Can you work these out from the model? Positions are in its coordinate system, mm. Face numbers are marked on the shaded views. A direction names the side the tool comes from. Round coordinates to 2 decimals unless told otherwise and drop trailing zeros. Write each loop counter-clockwise with the first axis right and the second up, starting at its lowest first coordinate (ties: lowest second). Pieces come first, ordered by that corner, then holes. Notation, with made-up numbers: (56, 33) -> (73, 33) arc R16 ccw to (73, 55) -> close; hole circle Ø6 at (77.25, 4). An arc over 180 degrees is marked (long way). Use CSV: the item, a comma, the result in double quotes.
```python
from build123d import *

# Parameters (mm, degrees)
SALIENTE_EXTRUIR1_DEPTH      = 77.5
SALIENTE_EXTRUIR1_DEPTH_BACK = 77.5
CROQUIS3_W                   = 82.87
CROQUIS3_H                   = 362
CROQUIS4_W                   = 230
CROQUIS4_H                   = 315.74
CROQUIS4_R                   = 110
SALIENTE_EXTRUIR2_DEPTH      = 495.3
CORTAR_EXTRUIR1_DEPTH        = 447.936166471
CORTAR_EXTRUIR1_DEPTH_BACK   = 447.936166471
CROQUIS5_W                   = 42
CROQUIS5_H                   = 360
CROQUIS6_W                   = 140.888518715
CROQUIS6_H                   = 52
CROQUIS6_W_2                 = 161.625356967
CORTAR_EXTRUIR2_DEPTH        = 332
CORTAR_EXTRUIR3_START        = -495.3
CORTAR_EXTRUIR3_DEPTH        = 495.3
CROQUIS12_R                  = 9.525
CORTAR_EXTRUIR9_DEPTH        = 230
CROQUIS15_R                  = 14.29
CORTAR_EXTRUIR10_DEPTH       = 48
CORTAR_EXTRUIR11_START       = -48
CROQUIS16_R                  = 14.29
CORTAR_EXTRUIR11_DEPTH       = 48
CROQUIS18_W                  = 231.274148036
CROQUIS18_H                  = 332
CORTAR_EXTRUIR12_DEPTH       = 48
CROQUIS19_W                  = 231.274148036
CROQUIS19_H                  = 332
CORTAR_EXTRUIR13_DEPTH       = 48
CROQUIS20_W                  = 52.279992223
CROQUIS20_H                  = 50
CORTAR_EXTRUIR14_DEPTH       = 48
CROQUIS21_W                  = 52.279992223
CROQUIS21_H                  = 50
CORTAR_EXTRUIR15_DEPTH       = 48


with BuildPart() as part:
    # Croquis1 → Revolución1 (revolve)
    with BuildSketch(Plane.XY, mode=Mode.PRIVATE) as revoluci_n1_sk:
        Polygon((-110, 93.3), (-105, 93.3), (-51.5, 0), (-51.5, -362), (-105, -402), (-110, -402), align=None)
    revolve(revoluci_n1_sk.sketch.rotate(Axis((0, 0, 0), (0, 1, 0)), 270), axis=Axis((0, 0, 0), (0, 1, 0)))

    # Croquis3 → Saliente-Extruir1 (add, two sides: drawn at the far end of the back side and taken through both)
    with BuildSketch(Plane(origin=(0, 0, 0), x_dir=(0, 0, -1), z_dir=(1, 0, 0)).offset(-SALIENTE_EXTRUIR1_DEPTH_BACK)):
        with Locations((116.435, -181)):
            Rectangle(CROQUIS3_W, CROQUIS3_H)
        with Locations((-116.435, -181)):
            Rectangle(CROQUIS3_W, CROQUIS3_H)
    extrude(amount=SALIENTE_EXTRUIR1_DEPTH + SALIENTE_EXTRUIR1_DEPTH_BACK)

    # Croquis4 → Saliente-Extruir2 (add)
    with BuildSketch(Plane(origin=(0, 93.3, 0), x_dir=(1, 0, 0), z_dir=(0, 1, 0))):
        Rectangle(CROQUIS4_W, CROQUIS4_H)
        Circle(CROQUIS4_R, mode=Mode.SUBTRACT)
    extrude(amount=-SALIENTE_EXTRUIR2_DEPTH)

    # Croquis5 → Cortar-Extruir1 (cut, two sides: drawn at the far end of the back side and taken through both)
    with BuildSketch(Plane.XY.offset(-CORTAR_EXTRUIR1_DEPTH_BACK)):
        with Locations((0, -180)):
            Rectangle(CROQUIS5_W, CROQUIS5_H)
    extrude(amount=CORTAR_EXTRUIR1_DEPTH + CORTAR_EXTRUIR1_DEPTH_BACK, mode=Mode.SUBTRACT)

    # Croquis6 → Cortar-Extruir2 (cut)
    with BuildSketch(Plane(origin=(0, 0, 0), x_dir=(1, 0, 0), z_dir=(0, 1, 0))):
        with Locations((-100.594259358, -3)):
            Rectangle(CROQUIS6_W, CROQUIS6_H)
        with Locations((110.962678484, 3)):
            Rectangle(CROQUIS6_W_2, CROQUIS6_H)
    extrude(amount=-CORTAR_EXTRUIR2_DEPTH, mode=Mode.SUBTRACT)

    # Croquis7 → Cortar-Extruir3 (cut)
    with BuildSketch(Plane(origin=(0, 93.3, 0), x_dir=(1, 0, 0), z_dir=(0, 1, 0)).offset(CORTAR_EXTRUIR3_START)):
        Polygon((-115, 157.87), (-57.5, 157.87), (-57.5, 115.637074018), (-115, 53.01), align=None)
        Polygon((57.5, 115.637074018), (57.5, 157.87), (115, 157.87), (115, 53.01), align=None)
        Polygon((115, -157.87), (57.5, -157.87), (57.5, -115.637074018), (115, -53.01), align=None)
        Polygon((-57.5, -115.637074018), (-57.5, -157.87), (-115, -157.87), (-115, -53.01), align=None)
    extrude(amount=CORTAR_EXTRUIR3_DEPTH, mode=Mode.SUBTRACT)

    # Croquis12 → Cortar-Extruir9 (cut)
    with BuildSketch(Plane.ZY.offset(115)):
        with Locations(Location((-90.237074018, -327.07, 0), (0, 0, 90))):
            Circle(CROQUIS12_R)
        with Locations(Location((-90.237074018, -35.052, 0), (0, 0, 90))):
            Circle(CROQUIS12_R)
        with Locations(Location((90.237074018, -35.052, 0), (0, 0, 270))):
            Circle(CROQUIS12_R)
        with Locations(Location((90.237074018, -327.07, 0), (0, 0, 270))):
            Circle(CROQUIS12_R)
    extrude(amount=-CORTAR_EXTRUIR9_DEPTH, mode=Mode.SUBTRACT)

    # Croquis15 → Cortar-Extruir10 (cut)
    with BuildSketch(Plane.ZY.offset(115)):
        with Locations((-90.237074018, -35.052)):
            Circle(CROQUIS15_R)
        with Locations((90.237074018, -35.052)):
            Circle(CROQUIS15_R)
        with Locations((90.237074018, -327.07)):
            Circle(CROQUIS15_R)
        with Locations((-90.237074018, -327.07)):
            Circle(CROQUIS15_R)
    extrude(amount=-CORTAR_EXTRUIR10_DEPTH, mode=Mode.SUBTRACT)

    # Croquis16 → Cortar-Extruir11 (cut)
    with BuildSketch(Plane(origin=(115, 0, 0), x_dir=(0, 0, -1), z_dir=(1, 0, 0)).offset(CORTAR_EXTRUIR11_START)):
        with Locations(Location((-90.237074018, -35.052, 0), (0, 0, 180))):
            Circle(CROQUIS16_R)
        with Locations(Location((90.237074018, -35.052, 0), (0, 0, 180))):
            Circle(CROQUIS16_R)
        with Locations(Location((90.237074018, -327.07, 0), (0, 0, 180))):
            Circle(CROQUIS16_R)
        with Locations(Location((-90.237074018, -327.07, 0), (0, 0, 180))):
            Circle(CROQUIS16_R)
    extrude(amount=CORTAR_EXTRUIR11_DEPTH, mode=Mode.SUBTRACT)

    # Croquis18 → Cortar-Extruir12 (cut)
    with BuildSketch(Plane(origin=(115, 0, 0), x_dir=(0, 0, -1), z_dir=(1, 0, 0))):
        with Locations((0, -166)):
            Rectangle(CROQUIS18_W, CROQUIS18_H)
    extrude(amount=-CORTAR_EXTRUIR12_DEPTH, mode=Mode.SUBTRACT)

    # Croquis19 → Cortar-Extruir13 (cut)
    with BuildSketch(Plane.ZY.offset(115)):
        with Locations((0, -166)):
            Rectangle(CROQUIS19_W, CROQUIS19_H)
    extrude(amount=-CORTAR_EXTRUIR13_DEPTH, mode=Mode.SUBTRACT)

    # Croquis20 → Cortar-Extruir14 (cut)
    with BuildSketch(Plane.ZY.offset(115)):
        with Locations((-79.149996112, 25)):
            Rectangle(CROQUIS20_W, CROQUIS20_H)
        with Locations((79.149996112, 25)):
            Rectangle(CROQUIS20_W, CROQUIS20_H)
    extrude(amount=-CORTAR_EXTRUIR14_DEPTH, mode=Mode.SUBTRACT)

    # Croquis21 → Cortar-Extruir15 (cut)
    with BuildSketch(Plane(origin=(115, 0, 0), x_dir=(0, 0, -1), z_dir=(1, 0, 0))):
        with Locations((79.149996112, 25)):
            Rectangle(CROQUIS21_W, CROQUIS21_H)
        with Locations((-79.149996112, 25)):
            Rectangle(CROQUIS21_W, CROQUIS21_H)
    extrude(amount=-CORTAR_EXTRUIR15_DEPTH, mode=Mode.SUBTRACT)


solid = part.part
```
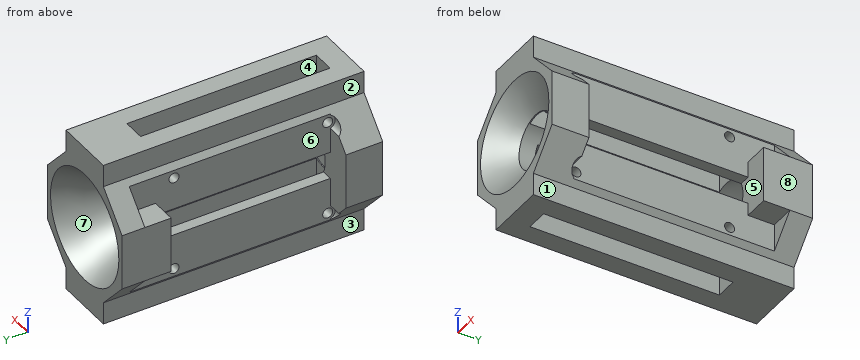
Q1. Suppose I cut it at A-A (y = -204.5). Write out the boundary of the cut face in (x, z).
Resolved:
outline,"(-67, -105.29) -> (-57.5, -115.64) -> (-57.5, -157.87) -> (-21, -157.87) -> (-21, -47.02) arc R51.5 cw to (-46.08, -23) -> (-67, -23) -> close; (-67, 29) -> (-42.56, 29) arc R51.5 cw to (-21, 47.02) -> (-21, 157.87) -> (-57.5, 157.87) -> (-57.5, 115.64) -> (-67, 105.29) -> close; (21, -157.87) -> (57.5, -157.87) -> (57.5, -115.64) -> (67, -105.29) -> (67, -29) -> (42.56, -29) arc R51.5 cw to (21, -47.02) -> close; (21, 47.02) arc R51.5 cw to (46.08, 23) -> (67, 23) -> (67, 105.29) -> (57.5, 115.64) -> (57.5, 157.87) -> (21, 157.87) -> close"
Q2. Will these pins go through, and if not, where does the flat tip stop? P1, Ø21, axis at y = -121, z = 143.5, coming from the +X side; P2, Ø8, axis at y = -90, z = 59.5, coming from the -X side; P3, Ø5, axis at x = 81.5, z = -28, coming from the -Y side.
Resolved:
P1,"stops at x = 57.5"
P2,"stops at x = -67"
P3,"stops at y = -389.79"
Q3. On a 3-axis mill with a long thin cutter (end or side, diameter ignored), from which of +Z, -Z, +X, -X, +Y, -Y can I reach the whole of each face in a straight line? I mean the marked faces 1, 2, 3, 4 and 5. Say none if no direction works.
Resolved:
face 1,"-Z, +X, +Y, -Y"
face 2,"+Z, -X, +Y, -Y"
face 3,"-Z, -X, +Y, -Y"
face 4,"+Z, -Z"
face 5,"+X"
Q4. Suppose I cut it at C-C (z = 0). Write out the boundary of the cut face in (x, y).
Resolved:
outline,"(-115, -402) -> (-105, -402) -> (-51.5, -362) -> (-51.5, -332) -> (-115, -332) -> close; (-115, 0) -> (-51.5, 0) -> (-105, 93.3) -> (-115, 93.3) -> close; (51.5, -362) -> (105, -402) -> (115, -402) -> (115, -332) -> (51.5, -332) -> close; (51.5, 0) -> (115, 0) -> (115, 93.3) -> (105, 93.3) -> close"
Q5. If we mould it in two halves opening along X, with no side actions, what happens to the marked faces 6, 7 and 8? For each: released by +X, released by -X, zero draft, split by the parting line, or undercut.
Resolved:
face 6,"released by -X"
face 7,"undercut"
face 8,"released by +X"
Q6. Suppose I cut it at B-B (x = 0). Write out the boundary of the cut face in (y, z).
Resolved:
outline,"(-402, -157.87) -> (-360, -157.87) -> (-360, -51.5) -> (-362, -51.5) -> (-402, -105) -> close; (-402, 105) -> (-362, 51.5) -> (-360, 51.5) -> (-360, 157.87) -> (-402, 157.87) -> close; (0, -157.87) -> (93.3, -157.87) -> (93.3, -105) -> (0, -51.5) -> close; (0, 51.5) -> (93.3, 105) -> (93.3, 157.87) -> (0, 157.87) -> close"
Q7. Please list where these lines run through material, in increasing order: probe 1 along Z at (x, y) = (56.5, -327.07); probe 2 along X at (y, z) = (-58, -93.5); probe 3 along Z at (x, y) = (48, -160.5).
Resolved:
probe 1,"z = -157.87 to -99.76, -80.71 to -29, 23 to 80.71, 99.76 to 157.87"
probe 2,"x = -67 to -21, 21 to 67"
probe 3,"z = -157.87 to -29, 23 to 157.87"
